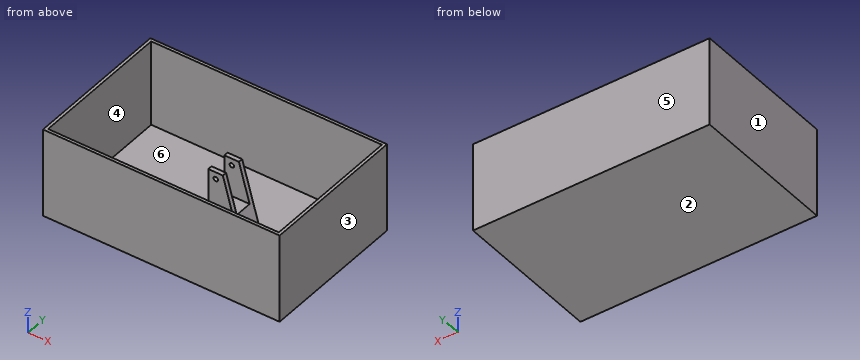
from build123d import *

# Parameters (mm, degrees)
F0_W     = 160
F0_H     = 100
F2_DEPTH = 60
F3_T     = -2
F4_R     = 1.5
F5_DEPTH = 9
F6_W     = 66.8862648116
F6_H     = 12
F7_DEPTH = 26


with BuildPart() as f2:
    # F0 (on Top) → F2 (new body)
    with BuildSketch(Plane.XY):
        Rectangle(F0_W, F0_H)
    extrude(amount=F2_DEPTH)

    # F3
    f3_openings = [f2.faces().sort_by_distance(p)[0] for p in [
        (0, 0, 60),
    ]]
    offset(amount=F3_T, openings=f3_openings)

    # F4 (on Front) → F5 (join, symmetric)
    with BuildSketch(Plane.XZ):
        Polygon((1.976594096, 44.2819991666), (1.976594096, 0), (24.1503274081, 0), (11.8152030863, 44.2819991666), align=None)
        with Locations((7.0080704532, 39.5950130723)):
            Circle(F4_R, mode=Mode.SUBTRACT)
    extrude(amount=F5_DEPTH, both=True)

    # F6 (on face) → F7 (cut)
    with BuildSketch(Plane.XY.offset(44.2819991666)):
        with Locations((3.9056837824, 0)):
            Rectangle(F6_W, F6_H)
    extrude(amount=-F7_DEPTH, mode=Mode.SUBTRACT)


solid = f2.part
Work out the finished part from the listing and answer in its coordinate system (mm). Face numbers are marked on the shaded views. A direction names the side the tool comes from. Round coordinates to 2 decimals unless told otherwise and drop trailing zeros. Write each loop counter-clockwise with the first axis right and the second up, starting at its lowest first coordinate (ties: lowest second). Pieces come first, ordered by that corner, then holes. Notation, with made-up numbers: (83, 11.5) - (131, 11.5) arc R17 ccw to (131, 28.5) - close; hole circle Ø1 at (44.25, 33.5). An arc over 180 degrees is marked (long way). Answer in a Markdown table with one row per item. Add a question column.
1. A cutting plane is placed at A-A, the plane z = 14. Determine the outline of the cut face in (x, y).
2. A cutting plane is placed at C-C, the plane x = -44.5. Determine the outline of the cut face in (y, z).
3. Given pin 1 (10 mm diameter, centred on x = 8.5, y = -39.5, fed in from -Z); pin 2 (10 mm diameter, centred on x = -1.5, y = 1.5, fed in from +Z); pin 3 (3.5 mm diameter, centred on x = 5.5, y = 7.5, fed in from +Z); pin 4 (4 mm diameter, centred on x = 53, y = 0.5, fed in from +Z), each flat-ended and moving along its own axis, determine where each tip first touches the part or whether it passes through.
4. A cutting plane is placed at D-D, the plane y = -25. Determine the outline of the cut face in (x, z), and give its area (3 significant figures).
5. A cutting plane is placed at B-B, the plane z = 32.5. Determine the outline of the cut face in (x, y), and give its area (3 significant figures).
6. Find the intervals of material crossed by line 1 along Y through (x, z) = (2.5, 2.5); line 2 along Y through (x, z) = (-49, 46); line 3 along X through (y, z) = (-39, 28), in increasing order. Write a range as from..to.
7. The mould has two halves that part along X. Classify the marked faces 1, 2, 3 and 4: +X half, -X half, draft (parallel to the pull), parting line (faces both ways), or undercut.
8. For the marked faces 5 and 6, determine the directions among +Z, -Z, +X, -X, +Y, -Y from which every point of the face is accessible in a straight line to the end or side of a thin tool.
Worked out:
| question | item | result |
|---|---|---|
| 1 | outline | (-80, -50) - (80, -50) - (80, 50) - (-80, 50) - close; (1.98, -9) - (20.25, -9) - (20.25, 9) - (1.98, 9) - close; hole (-78, -48) - (78, -48) - (78, 48) - (-78, 48) - close |
| 2 | outline | (-50, 0) - (50, 0) - (50, 60) - (48, 60) - (48, 2) - (-48, 2) - (-48, 60) - (-50, 60) - close |
| 3 | pin 1 | z = 0 |
| 3 | pin 2 | z = 18.28 |
| 3 | pin 3 | z = 44.28 |
| 3 | pin 4 | z = 2 |
| 4 | outline | (-80, 0) - (80, 0) - (80, 60) - (78, 60) - (78, 2) - (-78, 2) - (-78, 60) - (-80, 60) - close |
| 4 | area | 552 mm^2 |
| 5 | outline | (-80, -50) - (80, -50) - (80, 50) - (-80, 50) - close; (1.98, -9) - (15.1, -9) - (15.1, -6) - (1.98, -6) - close; (1.98, 6) - (15.1, 6) - (15.1, 9) - (1.98, 9) - close; hole (-78, -48) - (78, -48) - (78, 48) - (-78, 48) - close |
| 5 | area | 1,100 mm^2 |
| 6 | line 1 | -50..-48, -9..9, 48..50 |
| 6 | line 2 | -50..-48, 48..50 |
| 6 | line 3 | -80..-78, 78..80 |
| 7 | face 1 | -X half |
| 7 | face 2 | draft |
| 7 | face 3 | +X half |
| 7 | face 4 | undercut |
| 8 | face 5 | +Z, -Z, +X, -X, +Y |
| 8 | face 6 | +Z |
